from build123d import *

# Parameters (mm, degrees)
SKETCH_1_R               = 12
EXTRUDE_1_DEPTH          = 21
CUT_EXTRUDE_1_DEPTH      = 21
CUT_EXTRUDE_1_DEPTH_BACK = 21
HOLE_WIZARD_M20_2_D      = 17.5
CHAMFER_2_SIZE           = 1


with BuildPart() as part:
    # Sketch 1 → Extrude 1 (new body)
    with BuildSketch(Plane.XY):
        with Locations(Location((0, 0, 0), (0, 0, 180))):
            Circle(SKETCH_1_R)
    extrude(amount=EXTRUDE_1_DEPTH)

    # Sketch 2 → Cut-Extrude 1 (cut, two sides: drawn at the far end of the back side and taken through both)
    with BuildSketch(Plane(origin=(0, 0, 0), x_dir=(0, 0, -1), z_dir=(1, 0, 0)).offset(-CUT_EXTRUDE_1_DEPTH_BACK)):
        with BuildLine():
            Line((-21, 12), (-12.451705037, 1.058681393))
            ThreePointArc((-12.451705037, 1.058681393), (-8.852121463, -5.034581824), (-7.6, -12))
            Line((-7.6, -12), (-21, -12))
            Line((-21, -12), (-21, 12))
        make_face()
    extrude(amount=CUT_EXTRUDE_1_DEPTH + CUT_EXTRUDE_1_DEPTH_BACK, mode=Mode.SUBTRACT)

    # Hole Wizard M20 _2 (through all)
    with Locations(Plane(origin=(0, 0, 0), x_dir=(-1, 0, 0), z_dir=(0, 0, -1))):
        with Locations((0, 0)):
            Hole(HOLE_WIZARD_M20_2_D / 2)

    # Chamfer 2
    chamfer_2_edges = [part.edges().sort_by_distance(p)[0] for p in [
        (12, 0, 0),
    ]]
    chamfer(chamfer_2_edges, length=CHAMFER_2_SIZE)


solid = part.part
For this review, take the finished solid that the model builds, in its own axes (mm). Give positions to 0.01 mm unless a question says otherwise; leave off trailing zeros. Order: outer loops, then holes, each group sorted by start corner. A loop starts at its lowest first (then second) coordinate and runs counter-clockwise, first axis right, second up. Notation, with made-up numbers: (23, 34) - (50, 34) arc R13 ccw to (50, 49) - close; hole circle Ø9 at (2.25, -36.5). An arc over 180 degrees is marked (long way). Answer as a JSON object with one key per item and string values. Group by question number.
Item 1: Take a section at C-C on z = 15.25. Give the boundary of the cut face in (x, y), and give its area (3 significant figures).
Item 2: Draft analysis for pull direction X (two halves, no side actions). For faces 1 (the flat face through (-0.167, 9.037, 18.685)), 2 (the cylindrical face through (-1.139, 8.676, 7.309)), 3 (the cylindrical face through (2.601, 11.715, 8.638)), state which applies: pulls with the +X half, pulls with the -X half, needs draft (parallel to the pull), parting line crosses it, or undercut.
Item 3: Take a section at B-B on x = 0. Give the boundary of the cut face in (y, z), and give its area (3 significant figures).
Item 4: Take a section at A-A on y = 0. Give the boundary of the cut face in (x, z).
Item 5: Wall thickness on line 1 along Y through (x, z) = (0, 6.5); line 2 along X through (y, z) = (-7, 4); line 3 along Y through (x, z) = (0, 9.75): over which ranges is each line inside the solid? List them lowest first.
Item 6: Clearance check with flat-ended pins moving along their axes: pin 1 Ø10 at (x, y) = (0.5, 4) entering from +Z; pin 2 Ø5 at (x, z) = (5, 6) entering from +Y; pin 3 Ø4 at (x, z) = (-2, 12.5) entering from -Y. State where each tip first meets the part, or that it passes through.
Reported:
{
 "1": {"outline": "(-11.07, 4.64) - (-7.42, 4.64) arc R8.75 cw to (7.42, 4.64) - (11.07, 4.64) arc R12 ccw to start", "area": "74.6 mm^2"},
 "2": {"face 1": "needs draft", "face 2": "undercut", "face 3": "parting line crosses it"},
 "3": {"outline": "(-12, 1) - (-11, 0) - (-8.75, 0) - (-8.75, 7.87) arc R20 cw to (-12, 7.6) - close; (8.75, 0) - (11, 0) - (12, 1) - (12, 21) - (8.75, 18.46) - close", "area": "88.1 mm^2"},
 "4": {"outline": "(-12, 1) - (-11, 0) - (-8.75, 0) - (-8.75, 11.6) - (-12, 11.6) - close; (8.75, 0) - (11, 0) - (12, 1) - (12, 11.6) - (8.75, 11.6) - close"},
 "5": {"line 1": "-12 to -8.75, 8.75 to 12", "line 2": "-9.75 to -5.25, 5.25 to 9.75", "line 3": "8.75 to 12"},
 "6": {"pin 1": "z = 18.66", "pin 2": "y = 11.74", "pin 3": "y = 7.78"}
}
